```python
from build123d import *

# Parameters (mm, degrees)
BASPROSKE_W             = 5
BASPROSKE_H             = 4.25
TOOTHCUT_DEPTH          = 8.818247886
TEETHCUTS_COUNT         = 15
TEETHCUTS_ANGLE         = 336
BORSKE_R                = 0.5
BORE_DEPTH              = 50.0000508
SKETCH1_R               = 1.75
CUT_EXTRUDE1_DEPTH      = 8.811066965
CUT_EXTRUDE1_DEPTH_BACK = 8.811066965
SKETCH2_W               = 2
SKETCH2_H               = 1.1
CUT_EXTRUDE2_DEPTH      = 8.811066965
CUT_EXTRUDE2_DEPTH_BACK = 8.811066965


with BuildPart() as part:
    # BasProSke → Base-Revolve (revolve)
    with BuildSketch(Plane(origin=(0, 0, 0), x_dir=(1, 0, 0), z_dir=(0, 1, 0)), mode=Mode.PRIVATE) as base_revolve_sk:
        with Locations((2.5, 2.125)):
            Rectangle(BASPROSKE_W, BASPROSKE_H)
    revolve(base_revolve_sk.sketch.rotate(Axis((-10, 0, 0), (1, 0, 0)), 180), axis=Axis((-10, 0, 0), (1, 0, 0)))

    # TooCutSke → ToothCut (cut, through all)
    with BuildSketch(Plane(origin=(0, 0, 0), x_dir=(0, 0, -1), z_dir=(1, 0, 0))):
        with BuildLine():
            ThreePointArc((0.265767165, 3.112674704), (0, 3.124), (-0.265767165, 3.112674704))
            ThreePointArc((-0.265767165, 3.112674704), (-0.418628877, 3.712626775), (-0.800767345, 4.19974009))
            ThreePointArc((-0.800767345, 4.19974009), (0, 4.2754), (0.800767345, 4.19974009))
            ThreePointArc((0.800767345, 4.19974009), (0.418628877, 3.712626775), (0.265767165, 3.112674704))
        make_face()
    toothcut = extrude(amount=TOOTHCUT_DEPTH, mode=Mode.SUBTRACT)

    # TeethCuts: ToothCut ×15 about axis
    teethcuts_axis = Axis((-10, 0, 0), (1, 0, 0))
    for i in range(1, TEETHCUTS_COUNT):
        add(toothcut.rotate(teethcuts_axis, i * TEETHCUTS_ANGLE / (TEETHCUTS_COUNT - 1)), mode=Mode.SUBTRACT)

    # BorSke → Bore (cut, symmetric)
    with BuildSketch(Plane(origin=(0, 0, 0), x_dir=(0, 0, -1), z_dir=(1, 0, 0))):
        with Locations(Location((0, 0, 0), (0, 0, 180))):
            Circle(BORSKE_R)
    extrude(amount=BORE_DEPTH, both=True, mode=Mode.SUBTRACT)

    # Sketch1 → Cut-Extrude1 (cut, two sides)
    with BuildSketch(Plane(origin=(5, 0, 0), x_dir=(0, 0, -1), z_dir=(1, 0, 0))) as cut_extrude1_sk:
        Circle(SKETCH1_R)
    extrude(amount=CUT_EXTRUDE1_DEPTH, mode=Mode.SUBTRACT)
    extrude(cut_extrude1_sk.sketch, amount=-CUT_EXTRUDE1_DEPTH_BACK, mode=Mode.SUBTRACT)

    # Sketch2 → Cut-Extrude2 (cut, two sides)
    with BuildSketch(Plane(origin=(5, 0, 0), x_dir=(0, 0, -1), z_dir=(1, 0, 0))) as cut_extrude2_sk:
        with Locations((0, -1.75)):
            Rectangle(SKETCH2_W, SKETCH2_H)
    extrude(amount=CUT_EXTRUDE2_DEPTH, mode=Mode.SUBTRACT)
    extrude(cut_extrude2_sk.sketch, amount=-CUT_EXTRUDE2_DEPTH_BACK, mode=Mode.SUBTRACT)


solid = part.part
```
The model under review builds one solid part; all positions refer to its coordinate system, in mm. A direction names the side the tool comes from. Coordinates: 2 decimals unless noted, no trailing zeros. Order: outer loops, then holes, each group sorted by start corner. A loop starts at its lowest first (then second) coordinate and runs counter-clockwise, first axis right, second up. Notation, with made-up numbers: M 5,28 L 28,28 A9 cw 28,39 Z; hole C -6,54.5 d1. An arc over 180 degrees is marked long. One line per question, with ' | ' between items.
(1) The part is to be moulded in two halves that separate along Y. For faces 1 (the face through (2.46, 3.22, -1.89)), 2 (the face through (2.46, -3.54, 1.18)), 3 (the face through (2.465, -2.198, 2.992)), 4 (the face through (3, -2, -1)), say which applies: +Y half, -Y half, draft (parallel to the pull), parting line (faces both ways), or undercut.
Geometry results:
face 1: +Y half | face 2: -Y half | face 3: undercut | face 4: undercut
(2) For probe 1 along Z at (x, y) = (3.9, 3); probe 2 along Z at (x, y) = (2.8, 2); probe 3 along Y at (x, z) = (1.85, -3.5), list the stretches that pass through material, from the lowest coordinate up. Write a range as from..to.
Geometry results:
probe 1: z = -2.54..-1.68, -1.04..1.04, 1.68..2.54 | probe 2: z = -3.72..-2.65, -2.4..2.4, 2.65..3.72 | probe 3: y = -1.5..-0.72, -0.04..0.76, 1.65..2.23
(3) Add section C-C, the plane z = -3.5. Write out the cut boundary in (x, y).
Geometry results:
outline: M 0,-1.5 L 5,-1.5 L 5,-0.72 L 0,-0.72 Z; M 0,-0.04 L 5,-0.04 L 5,0.76 L 0,0.76 Z; M 0,1.65 L 5,1.65 L 5,2.23 L 0,2.23 Z
(4) Add section B-B, the plane y = 1. Write out the cut boundary in (x, z).
Geometry results:
outline: M 0,-2.96 L 5,-2.96 L 5,-1.44 L 0,-1.44 Z; M 0,1.44 L 5,1.44 L 5,2.96 L 0,2.96 Z
(5) Machinability: for faces 5 (the face through (2.46, 3.54, -1.13)), 6 (the face through (2.46, -2.75, 2.51)), 7 (the face through (2.465, 1.528, -3.384)), which of the approach directions +Z, -Z, +X, -X, +Y, -Y give a long, thin tool a straight path to every point of the face, cutting with its end or side? Answer none if there is none.
Geometry results:
face 5: +X, -X | face 6: +X, -X, -Y | face 7: -Z, +X, -X
(6) Add section A-A, the plane z = 0. Write out the cut boundary in (x, y), then the cut area to 3 significant figures.
Geometry results:
outline: M 0,-4.25 L 5,-4.25 L 5,-2.3 L 0,-2.3 Z; M 0,1.75 L 5,1.75 L 5,3.12 L 0,3.12 Z | area: 16.6 mm²
(7) Insertion check: pin 1 (3 mm diameter, centred on x = 1, y = 3, fed in from +Z); pin 2 (0.7 mm diameter, centred on x = 1.5, y = -2, fed in from -Z). Each pin has a flat end and moves straight along its axis. Give the tip position at first contact, or say it passes through.
Geometry results:
pin 1: stops at z = 3.73 | pin 2: stops at z = -3.08
